```python
from build123d import *

# Parameters (mm, degrees)
BASE_FLANGE1_DEPTH      = 11.25
SKETCH7_R               = 0.75
CUT_EXTRUDE1_DEPTH      = 24.598199084
SKETCH9_R               = 0.875
CUT_EXTRUDE2_DEPTH      = 16.790127454
FILL_START              = -0.75
FILL_PATTERN1_OUTLINE_R = 0.875
FILL_PATTERN1_DEPTH     = 0.75


# Read off the part's stored shape, not the designer's step: Fill Pattern1
# Sheet-metal steps are written as plain solids
with BuildPart() as part:
    # Sketch1 → Base-Flange1 (new, symmetric)
    with BuildSketch(Plane.XY):
        with BuildLine():
            Line((-10.125, -4.5), (-10.125, -0.85))
            ThreePointArc((-10.125, -0.85), (-9.876040764, -0.248959236), (-9.275, 0))
            Line((-9.275, 0), (9.275, 0))
            ThreePointArc((9.275, 0), (9.876040764, -0.248959236), (10.125, -0.85))
            Line((10.125, -0.85), (10.125, -4.5))
            Line((10.125, -4.5), (9.375, -4.5))
            Line((9.375, -4.5), (9.375, -0.85))
            ThreePointArc((9.375, -0.85), (9.345710678, -0.779289322), (9.275, -0.75))
            Line((9.275, -0.75), (-9.275, -0.75))
            ThreePointArc((-9.275, -0.75), (-9.345710678, -0.779289322), (-9.375, -0.85))
            Line((-9.375, -0.85), (-9.375, -4.5))
            Line((-9.375, -4.5), (-10.125, -4.5))
        make_face()
    extrude(amount=BASE_FLANGE1_DEPTH, both=True)

    # Sketch7 → Cut-Extrude1 (cut, through all)
    with BuildSketch(Plane(origin=(10.125, 0, 0), x_dir=(0, 0, -1), z_dir=(1, 0, 0))):
        with BuildLine():
            Line((-6.25, -1.35), (-6.25, -2))
            ThreePointArc((-6.25, -2), (-6.982233047, -3.767766953), (-8.75, -4.5))
            Line((-8.75, -4.5), (8.749999987, -4.5))
            ThreePointArc((8.749999987, -4.5), (6.982233042, -3.767766948), (6.25, -2))
            Line((6.25, -2), (6.25, -1.35))
            Line((6.25, -1.35), (-6.25, -1.35))
        make_face()
        with BuildLine():
            Line((-11.25, -4.5), (-8.75, -4.5))
            ThreePointArc((-8.75, -4.5), (-10.517766953, -3.767766953), (-11.25, -2))
            Line((-11.25, -2), (-11.25, -4.5))
        make_face()
        with BuildLine():
            ThreePointArc((11.25, -2), (10.517766948, -3.767766958), (8.749999987, -4.5))
            Line((8.749999987, -4.5), (11.25, -4.5))
            Line((11.25, -4.5), (11.25, -2))
        make_face()
        with Locations((8.75, -2)):
            Circle(SKETCH7_R)
        with Locations(Location((-8.75, -2, 0), (0, 0, 180))):
            Circle(SKETCH7_R)
    extrude(amount=-CUT_EXTRUDE1_DEPTH, mode=Mode.SUBTRACT)

    # Sketch9 → Cut-Extrude2 (cut, through all)
    with BuildSketch(Plane(origin=(0, 0, 0), x_dir=(1, 0, 0), z_dir=(0, 1, 0))):
        with Locations(Location((7.775, 9.5, 0), (0, 0, 180))):
            Circle(SKETCH9_R)
    extrude(amount=-CUT_EXTRUDE2_DEPTH, mode=Mode.SUBTRACT)

    # Fill Pattern1 outline → Fill Pattern1 (cut)
    with BuildSketch(Plane(origin=(0, 0, 0), x_dir=(1, 0, 0), z_dir=(0, 1, 0)).offset(FILL_START)):
        with Locations((-4.824497758, -9.413240898)):
            Circle(FILL_PATTERN1_OUTLINE_R)
        with Locations((-2.304598206, 6.590270631)):
            Circle(FILL_PATTERN1_OUTLINE_R)
        with Locations((-4.824497758, 8.045135316)):
            Circle(FILL_PATTERN1_OUTLINE_R)
        with Locations((-7.344397309, 9.5)):
            Circle(FILL_PATTERN1_OUTLINE_R)
        with Locations((7.775, 3.680541262)):
            Circle(FILL_PATTERN1_OUTLINE_R)
        with Locations((0.215301345, 5.135405947)):
            Circle(FILL_PATTERN1_OUTLINE_R)
        with Locations((2.735200897, 3.680541262)):
            Circle(FILL_PATTERN1_OUTLINE_R)
        with Locations((5.255100448, 2.225676578)):
            Circle(FILL_PATTERN1_OUTLINE_R)
        with Locations((7.775, 0.770811893)):
            Circle(FILL_PATTERN1_OUTLINE_R)
        with Locations((2.735200897, 9.5)):
            Circle(FILL_PATTERN1_OUTLINE_R)
        with Locations((5.255100448, 8.045135316)):
            Circle(FILL_PATTERN1_OUTLINE_R)
        with Locations((7.775, 6.590270631)):
            Circle(FILL_PATTERN1_OUTLINE_R)
        with Locations((-2.304598206, 9.5)):
            Circle(FILL_PATTERN1_OUTLINE_R)
        with Locations((0.215301345, 8.045135316)):
            Circle(FILL_PATTERN1_OUTLINE_R)
        with Locations((2.735200897, 6.590270631)):
            Circle(FILL_PATTERN1_OUTLINE_R)
        with Locations((5.255100448, 5.135405947)):
            Circle(FILL_PATTERN1_OUTLINE_R)
        with Locations((7.775, -7.958376213)):
            Circle(FILL_PATTERN1_OUTLINE_R)
        with Locations((-7.344397309, -2.138917475)):
            Circle(FILL_PATTERN1_OUTLINE_R)
        with Locations((-4.824497758, -3.59378216)):
            Circle(FILL_PATTERN1_OUTLINE_R)
        with Locations((-2.304598206, -5.048646844)):
            Circle(FILL_PATTERN1_OUTLINE_R)
        with Locations((5.255100448, -6.503511529)):
            Circle(FILL_PATTERN1_OUTLINE_R)
        with Locations((2.735200897, -5.048646844)):
            Circle(FILL_PATTERN1_OUTLINE_R)
        with Locations((0.215301345, -3.59378216)):
            Circle(FILL_PATTERN1_OUTLINE_R)
        with Locations((-2.304598206, -2.138917475)):
            Circle(FILL_PATTERN1_OUTLINE_R)
        with Locations((-4.824497758, -6.503511529)):
            Circle(FILL_PATTERN1_OUTLINE_R)
        with Locations((-2.304598206, -7.958376213)):
            Circle(FILL_PATTERN1_OUTLINE_R)
        with Locations((0.215301345, -9.413240898)):
            Circle(FILL_PATTERN1_OUTLINE_R)
        with Locations((-7.344397309, -7.958376213)):
            Circle(FILL_PATTERN1_OUTLINE_R)
        with Locations((0.215301345, -6.503511529)):
            Circle(FILL_PATTERN1_OUTLINE_R)
        with Locations((2.735200897, -7.958376213)):
            Circle(FILL_PATTERN1_OUTLINE_R)
        with Locations((5.255100448, -9.413240898)):
            Circle(FILL_PATTERN1_OUTLINE_R)
        with Locations((-7.344397309, -5.048646844)):
            Circle(FILL_PATTERN1_OUTLINE_R)
        with Locations((2.735200897, 0.770811893)):
            Circle(FILL_PATTERN1_OUTLINE_R)
        with Locations((5.255100448, -0.684052791)):
            Circle(FILL_PATTERN1_OUTLINE_R)
        with Locations((7.775, -2.138917475)):
            Circle(FILL_PATTERN1_OUTLINE_R)
        with Locations((-7.344397309, 3.680541262)):
            Circle(FILL_PATTERN1_OUTLINE_R)
        with Locations((0.215301345, 2.225676578)):
            Circle(FILL_PATTERN1_OUTLINE_R)
        with Locations((-2.304598206, 3.680541262)):
            Circle(FILL_PATTERN1_OUTLINE_R)
        with Locations((-4.824497758, 5.135405947)):
            Circle(FILL_PATTERN1_OUTLINE_R)
        with Locations((-7.344397309, 6.590270631)):
            Circle(FILL_PATTERN1_OUTLINE_R)
        with Locations((-4.824497758, -0.684052791)):
            Circle(FILL_PATTERN1_OUTLINE_R)
        with Locations((-7.344397309, 0.770811893)):
            Circle(FILL_PATTERN1_OUTLINE_R)
        with Locations((7.775, -5.048646844)):
            Circle(FILL_PATTERN1_OUTLINE_R)
        with Locations((5.255100448, -3.59378216)):
            Circle(FILL_PATTERN1_OUTLINE_R)
        with Locations((2.735200897, -2.138917475)):
            Circle(FILL_PATTERN1_OUTLINE_R)
        with Locations((0.215301345, -0.684052791)):
            Circle(FILL_PATTERN1_OUTLINE_R)
        with Locations((-2.304598206, 0.770811893)):
            Circle(FILL_PATTERN1_OUTLINE_R)
        with Locations((-4.824497758, 2.225676578)):
            Circle(FILL_PATTERN1_OUTLINE_R)
    extrude(amount=FILL_PATTERN1_DEPTH, mode=Mode.SUBTRACT)


solid = part.part
```
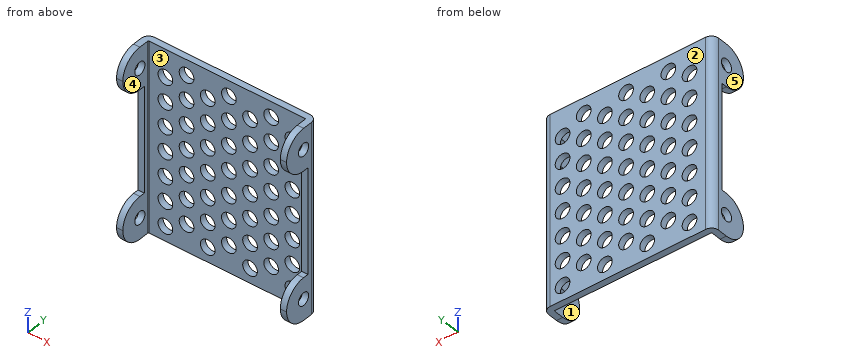
Can you work these out from the model? Positions are in its coordinate system, mm. Face numbers are marked on the shaded views. A direction names the side the tool comes from. Coordinates: 2 decimals unless noted, no trailing zeros.
1. I need wall thicknesses on line 1 (X direction, y = -0.65, z = -1.75); line 2 (X direction, y = -2, z = -7.5) (3 decimals); line 3 (X direction, y = -0.45, z = -7.75) (3 decimals). Which ranges of each line are inside material? Lowest first, please.
2. I'm going to push a flat-ended pin straight in: pin 1 (2 mm diameter, centred on x = 5.26, z = -8.05, fed in from -Y). Where does the tip first touch, or does it pass through?
3. If we section it at A-A (y = -2.3): Give the number of separate pieces and of enclosed holes in the cut face, then the cut area to 3 significant figures.
4. Thinking about a two-plate mould opening in Y: for the marked faces 1, 2 and 3, which applies, +Y half, -Y half, draft (parallel to the pull), parting line (faces both ways), or undercut?
5. For the marked faces 4 and 5, which set-ups out of +Z, -Z, +X, -X, +Y, -Y let a thin tool reach every point of the face, with its end or its side?
Entries:
1. line 1: x = -10.1 to -5.56, -4.09 to -0.52, 0.95 to 4.52, 5.99 to 10.1
1. line 2: x = -10.125 to -9.375, 9.375 to 10.125
1. line 3: x = -10.025 to -5.648, -4.001 to -0.608, 1.039 to 4.431, 6.079 to 10.025
2. pin 1: stops at y = -0.75
3. separate pieces: 8
3. enclosed holes: 0
3. area: 10.8 mm2
4. face 1: draft
4. face 2: +Y half
4. face 3: -Y half
5. face 4: +Z, -Z, -Y
5. face 5: +Z, -Z, -X, +Y, -Y
